Could you check a few things on this model? Use its own coordinates, in mm. Face numbers are marked on the shaded views. A direction names the side the tool comes from. Give positions to 0.01 mm unless a question says otherwise; leave off trailing zeros. Loops run counter-clockwise (first coordinate to the right, second up) from the corner with the lowest first, then second, coordinate; pieces in that order, holes last. Notation, with made-up numbers: M -10.75,3.5 L 46.25,3.5 A19 ccw 46.25,26.5 Z; hole C -18.75,-13 d3. An arc over 180 degrees is marked long. Answer in a Markdown table with one row per item. Add a question column.
1. If we section it at C-C on x = 2.25: List the corners of the cut face in (y, z) for me, then the cut area to 3 significant figures.
2. I need wall thicknesses on line 1 along X through (y, z) = (1.45, 2.1); line 2 along Z through (x, y) = (4.25, -0.1); line 3 along Y through (x, z) = (9.5, 0.25). Which ranges of each line are inside material? Lowest first, please. Write a range as from..to.
3. Which directions (+Z, -Z, +X, -X, +Y, -Y) give clear straight access to the entire face, cutting with the end or side of a thin tool? Please do the marked faces 1, 2 and 3.
4. I'm going to push a flat-ended pin straight in: pin 1 Ø2.5 at (y, z) = (-1.5, -1.5) entering from -X. Where does the tip first touch, or does it pass through?
5. If we section it at A-A on y = 2: List the corners of the cut face in (x, z) for me, then the cut area to 3 significant figures.
6. If we section it at B-B on z = 2: List the corners of the cut face in (x, y) for me, then the cut area to 3 significant figures.
```python
from build123d import *

# Parameters (mm, degrees)
F0_R     = 2.5
F1_DEPTH = 10
F3_DEPTH = 2.5


with BuildPart() as f1:
    # F0 (on Right) → F1 (new body)
    with BuildSketch(Plane.YZ):
        Circle(F0_R)
    extrude(amount=F1_DEPTH)

    # F2 (on face) → F3 (join)
    with BuildSketch(Plane.YZ.offset(10)):
        with BuildLine():
            ThreePointArc((0, 2.5), (-1.767767, 1.767767), (-2.5, 0))
            ThreePointArc((-2.5, 0), (-1.767767, -1.767767), (0, -2.5))
            ThreePointArc((0, -2.5), (1.767767, -1.767767), (2.5, 0))
            ThreePointArc((2.5, 0), (1.767767, 1.767767), (0, 2.5))
        make_face()
        with BuildLine():
            Line((-2.5, 2.5), (-2.5, 0))
            ThreePointArc((-2.5, 0), (-1.767767, 1.767767), (0, 2.5))
            Line((0, 2.5), (-2.5, 2.5))
        make_face()
        with BuildLine():
            Line((2.814407, 2.5), (0, 2.5))
            ThreePointArc((0, 2.5), (1.767767, 1.767767), (2.5, 0))
            ThreePointArc((2.5, 0), (1.767767, -1.767767), (0, -2.5))
            Line((0, -2.5), (2.814407, -2.5))
            Line((2.814407, -2.5), (2.814407, 2.5))
        make_face()
        with BuildLine():
            ThreePointArc((0, -2.5), (-1.767767, -1.767767), (-2.5, 0))
            Line((-2.5, 0), (-2.5, -2.5))
            Line((-2.5, -2.5), (0, -2.5))
        make_face()
    extrude(amount=F3_DEPTH)


solid = f1.part
```
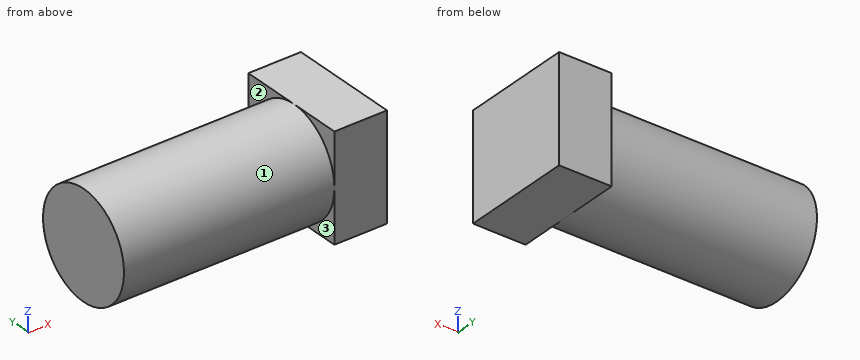
Results:
| question | item | result |
|---|---|---|
| 1 | outline | C 0,0 d5 |
| 1 | area | 19.6 mm2 |
| 2 | line 1 | 10..12.5 |
| 2 | line 2 | -2.5..2.5 |
| 2 | line 3 | -2.49..2.49 |
| 3 | face 1 | -X |
| 3 | face 2 | -X, +Y |
| 3 | face 3 | -Z, -X, -Y |
| 4 | pin 1 | x = 0 |
| 5 | outline | M 0,-1.5 L 10,-1.5 L 10,-2.5 L 12.5,-2.5 L 12.5,2.5 L 10,2.5 L 10,1.5 L 0,1.5 Z |
| 5 | area | 42.5 mm2 |
| 6 | outline | M 0,-1.5 L 10,-1.5 L 10,-2.5 L 12.5,-2.5 L 12.5,2.81 L 10,2.81 L 10,1.5 L 0,1.5 Z |
| 6 | area | 43.3 mm2 |
